Work out the finished part from the listing and answer in its coordinate system (mm). A direction names the side the tool comes from. Round coordinates to 2 decimals unless told otherwise and drop trailing zeros. Loops run counter-clockwise (first coordinate to the right, second up) from the corner with the lowest first, then second, coordinate; pieces in that order, holes last. Notation, with made-up numbers: (74, 62.25) - (93, 62.25) arc R15 ccw to (93, 83.25) - close; hole circle Ø2 at (-0.5, -16.75). An arc over 180 degrees is marked (long way). Answer as CSV lines item,"result". Start each with the question number.
Q1. For faces 1 (the face through (30, 4, 8.5)), 2 (the face through (0, 3, 56)), determine the directions among +Z, -Z, +X, -X, +Y, -Y from which every point of the face is accessible in a straight line to the end or side of a thin tool.
Q2. Straight lines are drawn through the part: L1, parallel to Z at x = 41, y = 5.5; L2, parallel to Z at x = 61, y = 9.75; L3, parallel to Y at x = 14, z = 4.5. For each, find the intervals that lie inside material, in ascending order. Write a range as [from, to].
Q3. Section D-D on x = 66 is taken. Write down the section's boundary in (y, z), then the cut area to 3 significant figures.
Q4. Section C-C on z = 30 is taken. Write down the section's boundary in (x, y).
Q5. This flat-tipped pin is pushed along its axis until it touches: pin 1 Ø1 at (y, z) = (7, 28.5) entering from -X. Where does it stop, or does it pass through?
Q6. Section A-A on y = 8.5 is taken. Write down the section's boundary in (x, z), then the cut area to 3 significant figures.
Q7. Section B-B on x = 78 is taken. Write down the section's boundary in (y, z), then the cut area to 3 significant figures.
Q8. The mould has two halves that part along Z. Classify faces 3 (the face through (90, 7, 30)), 4 (the face through (54, 6, 0)), 5 (the face through (30, 4, 51.5)): +Z half, -Z half, draft (parallel to the pull), parting line (faces both ways), or undercut.
Autodesk Fusion 360 part; units mm, degrees
sketch "Sketch1" plane through (0, 0, 0) normal (0, 0, 1) x (1, 0, 0)
  line L0 (0, 0) -> (90, 0)
  line L1 (90, 0) -> (90, 14)
  line L2 (90, 14) -> (0, 5)
  line L3 (0, 5) -> (0, 0)
  dimension "d1" = 5
  dimension "d2" = 14
  dimension "d3" = 90
extrude "Extrude1" add sketch "Sketch1" along normal blind 60
sketch "Sketch2" plane through (0, 0, 0) normal (0, -1, 0) x (1, 0, 0)
  line L0 (0, 0) -> (90, 0)
  line L1 (90, 0) -> (90, 60)
  line L2 (90, 60) -> (0, 60)
  line L3 (0, 60) -> (0, 0)
  line L4 (0, 30) -> (90, 30) construction
  line L5 (58.5, 51.5) -> (0, 51.5)
  line L6 (58.5, 8.5) -> (0, 8.5)
  arc A0 (58.5, 8.5) -> (58.5, 51.5) centre (58.5, 30) ccw
  dimension "d6" = 43
  dimension "d8" = 10
extrude "Extrude2" cut sketch "Sketch2" against normal blind 46.857 contours L3 L5 L6 A0
Findings:
1,face 1,"-X, +Y, -Y"
1,face 2,"+Z, -Z, -X, +Y, -Y"
2,L1,"z = [0, 8.5], [51.5, 60]"
2,L2,"z = [0, 8.65], [51.35, 60]"
2,L3,"y = [0, 6.4]"
3,outline,"(0, 0) - (11.6, 0) - (11.6, 9.85) - (0, 9.85) - close; (0, 50.15) - (11.6, 50.15) - (11.6, 60) - (0, 60) - close"
3,area,"229 mm^2"
4,outline,"(80, 0) - (90, 0) - (90, 14) - (80, 13) - close"
5,pin 1,"stops at x = 79.91"
6,outline,"(35, 0) - (90, 0) - (90, 60) - (35, 60) - (35, 51.5) - (58.5, 51.5) arc R21.5 cw to (58.5, 8.5) - (35, 8.5) - close"
6,area,"1,560 mm^2"
7,outline,"(0, 0) - (12.8, 0) - (12.8, 20.94) - (0, 20.94) - close; (0, 39.06) - (12.8, 39.06) - (12.8, 60) - (0, 60) - close"
7,area,"536 mm^2"
8,face 3,"draft"
8,face 4,"-Z half"
8,face 5,"undercut"
